Study the drawing (mm; zero at the part's minimum x, y, z) and answer. A direction names the side the tool comes from. Give positions to 0.01 mm unless a question says otherwise; leave off trailing zeros. Write each loop counter-clockwise with the first axis right and the second up, starting at its lowest first coordinate (ties: lowest second). Pieces come first, ordered by that corner, then holes.
1) A tool of negligible diameter and unlimited length cuts with its end or side. For the marked faces 4, 5, 6, 7 and 8, from which of +Z, -Z, +X, -X, +Y, -Y can it reach the whole face along a straight path? Write none if from no direction.
2) Straight lines are drawn through the part: probe 1 along Y at (x, z) = (4, 0.75); probe 2 along Z at (x, y) = (15.5, 34.5); probe 3 along X at (y, z) = (23, 63). For each, find the intervals that lie inside material, in ascending order.
3) Determine the mould class of the marked faces 1, 2 and 3 for opening direction X: pulls with the +X half, pulls with the -X half, needs draft (parallel to the pull), parting line crosses it, or undercut.
4) Find section B-B (z = 22.5). Determine the outline of the cut face in (x, y).
5) Given pin 1 Ø8 at (x, z) = (24, 37.5) entering from -Y; pin 2 Ø6 at (x, y) = (9, 45.5) entering from +Z; pin 3 Ø4 at (x, z) = (10.3, 13.5) entering from +Y; pin 4 Ø3 at (x, z) = (20.7, 63.5) entering from +Y, each flat-ended and moving along its own axis, determine where each tip first touches the part or whether it passes through.
6) Find section D-D (x = 14). Determine the outline of the cut face in (y, z), plus the area to 3 significant figures.
7) Find section C-C (y = 34.5). Determine the outline of the cut face in (x, z), plus the area to 3 significant figures.
8) Find section A-A (x = 20.7). Determine the outline of the cut face in (y, z).
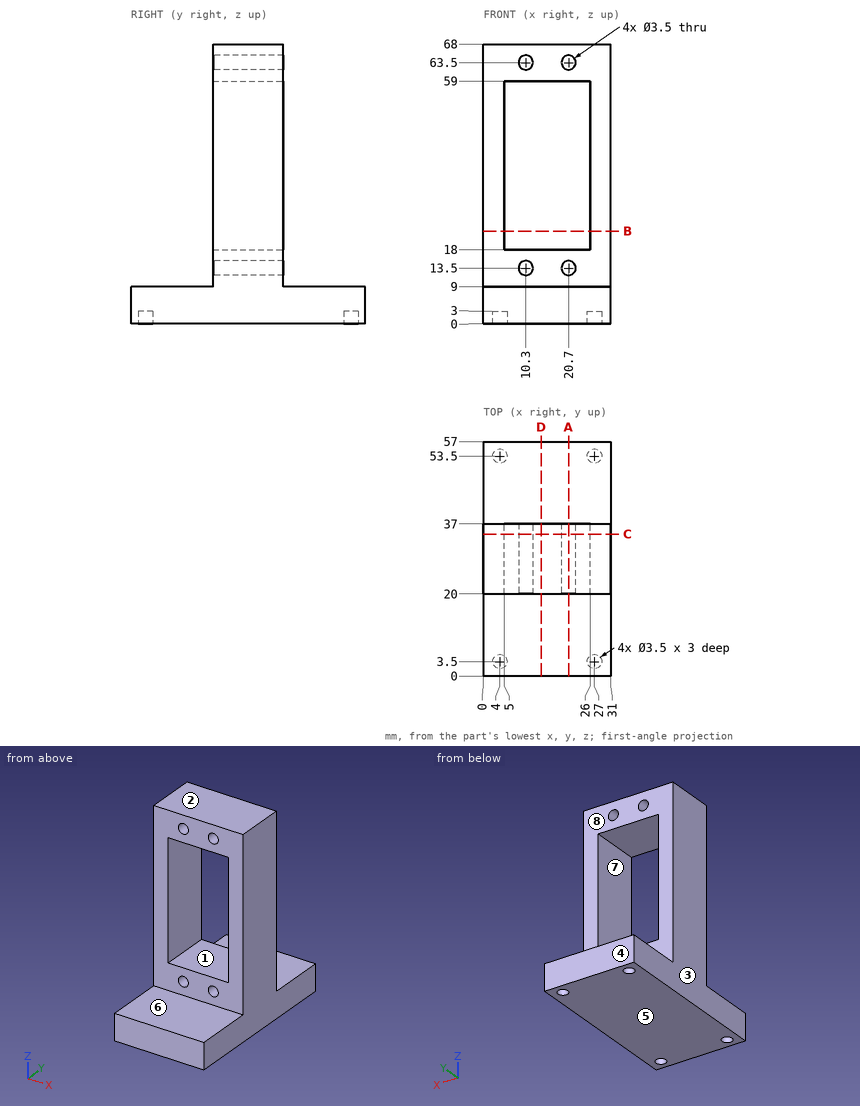
Results:
1. face 4: +Z, -Z, +X, -X, +Y
1. face 5: -Z, +X, -X, +Y, -Y
1. face 6: +Z, +X, -X, -Y
1. face 7: +Y, -Y
1. face 8: +Z, +X, -X, +Y
2. probe 1: y = 0 to 1.75, 5.25 to 51.75, 55.25 to 57
2. probe 2: z = 0 to 18, 59 to 68
2. probe 3: x = 0 to 8.62, 11.98 to 19.02, 22.38 to 31
3. face 1: undercut
3. face 2: needs draft
3. face 3: pulls with the -X half
4. outline: (0, 20) - (5, 20) - (5, 37) - (0, 37) - close; (26, 20) - (31, 20) - (31, 37) - (26, 37) - close
5. pin 1: stops at y = 20
5. pin 2: stops at z = 9
5. pin 3: stops at y = 37
5. pin 4: passes through
6. outline: (0, 0) - (57, 0) - (57, 9) - (37, 9) - (37, 18) - (20, 18) - (20, 9) - (0, 9) - close; (20, 59) - (37, 59) - (37, 68) - (20, 68) - close
6. area: 819 mm2
7. outline: (0, 0) - (31, 0) - (31, 68) - (0, 68) - close; hole (5, 18) - (26, 18) - (26, 59) - (5, 59) - close; hole circle Ø3.5 at (10.3, 13.5); hole circle Ø3.5 at (10.3, 63.5); hole circle Ø3.5 at (20.7, 13.5); hole circle Ø3.5 at (20.7, 63.5)
7. area: 1,210 mm2
8. outline: (0, 0) - (57, 0) - (57, 9) - (37, 9) - (37, 11.75) - (20, 11.75) - (20, 9) - (0, 9) - close; (20, 15.25) - (37, 15.25) - (37, 18) - (20, 18) - close; (20, 59) - (37, 59) - (37, 61.75) - (20, 61.75) - close; (20, 65.25) - (37, 65.25) - (37, 68) - (20, 68) - close
